Source: CAD feature listing. Evaluate the final solid. Frame: model axes, mm. A direction names the side the tool comes from. Round coordinates to 2 decimals unless told otherwise and drop trailing zeros. Loops run counter-clockwise (first coordinate to the right, second up) from the corner with the lowest first, then second, coordinate; pieces in that order, holes last. Notation, with made-up numbers: (58.5, 26) - (103.5, 26) arc R16 cw to (103.5, 49) - close; hole circle Ø11 at (89, 86.25). An arc over 180 degrees is marked (long way). One line per question, with ' | ' between items. Start each with the question number.
1. Ray query, line 1 (X direction, y = 49.5, z = -42.5); line 2 (Z direction, x = -52.5, y = 27.5); line 3 (Z direction, x = -27, y = 32.5). Return the intervals inside material, ascending.
2. Cut plane D-D (y = 68.5). Return loops of the section in (x, z).
3. Mould query, pull axis X, two halves, no side actions, for faces 1 (the flat face through (-1, 28, 45)), 2 (the cylindrical face through (-53.7, 27, 43.4)), 3 (the flat face through (0.7, 69.873, -42.465)). Classes: pulls with the +X half, pulls with the -X half, needs draft (parallel to the pull), parting line crosses it, or undercut.
4. Access query for faces 4 (the flat face through (-55, 27, -1)), 5 (the flat face through (-53, -19, 29)), 6 (the flat face through (50, 17, -1)), 7 (the flat face through (53, 57.5, 1)). Directions: +Z, -Z, +X, -X, +Y, -Y. A direction counts if a zero-diameter tool reaches every point of the face in a straight line with its end or side. Return the directions, or none.
5. Cut plane A-A (x = -52.5). Return loops of the section in (y, z), then the cut area to 3 significant figures.
6. Cut plane B-B (z = 17.5). Return loops of the section in (x, y), then the cut area to 3 significant figures.
7. Pin query (flat end, axial travel): pin 1 (4 mm diameter, centred on x = 53.5, z = 10, fed in from +Y); pin 2 (5.5 mm diameter, centred on x = -52, z = -3.5, fed in from -Y); pin 3 (1.7 mm diameter, centred on y = 59, z = -43.5, fed in from +X); pin 4 (5 mm diameter, centred on x = 52.5, z = 42.5, fed in from -Y). Return the tip coordinate at first contact, or that it passes through.
8. Cut plane C-C (y = -18). Return loops of the section in (x, z), then the cut area to 3 significant figures.
```python
from build123d import *

# Parameters (mm, degrees)
SKETCH1_W                = 100
SKETCH1_H                = 5
BOSS_EXTRUDE3_DEPTH      = 80
BOSS_EXTRUDE3_DEPTH_BACK = 24.960779397
SKETCH2_R                = 1.5
CUT_EXTRUDE1_DEPTH       = 80
SKETCH3_R                = 1.5
CUT_EXTRUDE2_DEPTH       = 80
SKETCH4_R                = 1.5
CUT_EXTRUDE3_DEPTH       = 80
SKETCH5_R                = 1.5
CUT_EXTRUDE4_DEPTH       = 80
CUT_EXTRUDE5_DEPTH       = 90
SKETCH7_W                = 90
SKETCH7_H                = 2.5
CUT_EXTRUDE7_DEPTH       = 5
CUT_EXTRUDE8_DEPTH       = 90
CUT_EXTRUDE11_DEPTH      = 90
SKETCH4_3_R              = 1.5
CUT_EXTRUDE17_DEPTH      = 105
SKETCH5_3_R              = 1.5
CUT_EXTRUDE18_DEPTH      = 105
SKETCH3_3_R              = 1.5
CUT_EXTRUDE19_DEPTH      = 105
SKETCH2_3_R              = 1.5
CUT_EXTRUDE20_DEPTH      = 105
SKETCH20_W               = 58
SKETCH20_H               = 13
CUT_EXTRUDE21_DEPTH      = 5


with BuildPart() as part:
    # Sketch1 → Boss-Extrude3 (new body, two sides)
    with BuildSketch(Plane(origin=(0, 0, 0), x_dir=(1, 0, 0), z_dir=(0, 1, 0))) as boss_extrude3_sk:
        with Locations((0, 42.5)):
            Rectangle(SKETCH1_W, SKETCH1_H)
        Polygon((-50, 45), (-55, 45), (-55, -45), (-50, -45), (-50, -40), (-50, 40), align=None)
        Polygon((55, 45), (50, 45), (50, 40), (50, -40), (50, -45), (55, -45), align=None)
        with Locations((0, -42.5)):
            Rectangle(SKETCH1_W, SKETCH1_H)
    extrude(amount=BOSS_EXTRUDE3_DEPTH)
    extrude(boss_extrude3_sk.sketch, amount=-BOSS_EXTRUDE3_DEPTH_BACK)

    # Sketch2 → Cut-Extrude1 (cut)
    with BuildSketch(Plane(origin=(0, 80, 0), x_dir=(1, 0, 0), z_dir=(0, 1, 0))):
        with Locations((-52.5, 42.5)):
            Circle(SKETCH2_R)
    extrude(amount=-CUT_EXTRUDE1_DEPTH, mode=Mode.SUBTRACT)

    # Sketch3 → Cut-Extrude2 (cut)
    with BuildSketch(Plane(origin=(0, 80, 0), x_dir=(1, 0, 0), z_dir=(0, 1, 0))):
        with Locations((52.5, 42.5)):
            Circle(SKETCH3_R)
    extrude(amount=-CUT_EXTRUDE2_DEPTH, mode=Mode.SUBTRACT)

    # Sketch4 → Cut-Extrude3 (cut)
    with BuildSketch(Plane(origin=(0, 80, 0), x_dir=(1, 0, 0), z_dir=(0, 1, 0))):
        with Locations((-52.5, -42.5)):
            Circle(SKETCH4_R)
    extrude(amount=-CUT_EXTRUDE3_DEPTH, mode=Mode.SUBTRACT)

    # Sketch5 → Cut-Extrude4 (cut)
    with BuildSketch(Plane(origin=(0, 80, 0), x_dir=(1, 0, 0), z_dir=(0, 1, 0))):
        with Locations((52.5, -42.5)):
            Circle(SKETCH5_R)
    extrude(amount=-CUT_EXTRUDE4_DEPTH, mode=Mode.SUBTRACT)

    # Sketch6 → Cut-Extrude5 (cut)
    with BuildSketch(Plane.XY.offset(45)):
        Polygon((-55, 80), (55, 80), (55, 60), align=None)
    extrude(amount=-CUT_EXTRUDE5_DEPTH, mode=Mode.SUBTRACT)

    # Sketch7 → Cut-Extrude7 (cut)
    with BuildSketch(Plane(origin=(55, 0, 0), x_dir=(0, 0, -1), z_dir=(1, 0, 0))):
        with Locations((0, 58.75)):
            Rectangle(SKETCH7_W, SKETCH7_H)
    extrude(amount=-CUT_EXTRUDE7_DEPTH, mode=Mode.SUBTRACT)

    # Sketch8 → Cut-Extrude8 (cut)
    with BuildSketch(Plane.XY.offset(45)):
        Polygon((50, 60), (55, 60), (50, 60.909090909), align=None)
    extrude(amount=-CUT_EXTRUDE8_DEPTH, mode=Mode.SUBTRACT)

    # Sketch9 → Cut-Extrude11 (cut)
    with BuildSketch(Plane.XY.offset(45)):
        Polygon((-55, 80), (-55, 77.5), (-50, 77.5), (-50, 79.090909091), align=None)
    extrude(amount=-CUT_EXTRUDE11_DEPTH, mode=Mode.SUBTRACT)

    # Sketch4_3 → Cut-Extrude17 (cut)
    with BuildSketch(Plane(origin=(0, 80, 0), x_dir=(1, 0, 0), z_dir=(0, 1, 0))):
        with Locations((-52.5, -42.5)):
            Circle(SKETCH4_3_R)
    extrude(amount=-CUT_EXTRUDE17_DEPTH, mode=Mode.SUBTRACT)

    # Sketch5_3 → Cut-Extrude18 (cut)
    with BuildSketch(Plane(origin=(0, 80, 0), x_dir=(1, 0, 0), z_dir=(0, 1, 0))):
        with Locations((52.5, -42.5)):
            Circle(SKETCH5_3_R)
    extrude(amount=-CUT_EXTRUDE18_DEPTH, mode=Mode.SUBTRACT)

    # Sketch3_3 → Cut-Extrude19 (cut)
    with BuildSketch(Plane(origin=(0, 80, 0), x_dir=(1, 0, 0), z_dir=(0, 1, 0))):
        with Locations((52.5, 42.5)):
            Circle(SKETCH3_3_R)
    extrude(amount=-CUT_EXTRUDE19_DEPTH, mode=Mode.SUBTRACT)

    # Sketch2_3 → Cut-Extrude20 (cut)
    with BuildSketch(Plane(origin=(0, 80, 0), x_dir=(1, 0, 0), z_dir=(0, 1, 0))):
        with Locations((-52.5, 42.5)):
            Circle(SKETCH2_3_R)
    extrude(amount=-CUT_EXTRUDE20_DEPTH, mode=Mode.SUBTRACT)

    # Sketch20 → Cut-Extrude21 (cut)
    with BuildSketch(Plane.ZY.offset(55)):
        with Locations((0, -18.460779397)):
            Rectangle(SKETCH20_W, SKETCH20_H)
    extrude(amount=-CUT_EXTRUDE21_DEPTH, mode=Mode.SUBTRACT)


solid = part.part
```
Answers follow:
1) line 1: x = -55 to -54, -51 to 51, 54 to 55 | line 2: z = -45 to -44, -41 to 41, 44 to 45 | line 3: z = -45 to -40, 40 to 45
2) outline: (-55, -45) - (8.25, -45) - (8.25, -40) - (-50, -40) - (-50, 40) - (8.25, 40) - (8.25, 45) - (-55, 45) - close; hole circle Ø3 at (-52.5, -42.5); hole circle Ø3 at (-52.5, 42.5)
3) face 1: needs draft | face 2: undercut | face 3: pulls with the +X half
4) face 4: +Z, -Z, -X, +Y, -Y | face 5: -X, -Y | face 6: +Y, -Y | face 7: +Z, -Z, +X, +Y
5) outline: (-24.96, -45) - (77.5, -45) - (77.5, -44) - (-24.96, -44) - close; (-24.96, -41) - (77.5, -41) - (77.5, 41) - (-24.96, 41) - (-24.96, 29) - (-11.96, 29) - (-11.96, -29) - (-24.96, -29) - close; (-24.96, 44) - (77.5, 44) - (77.5, 45) - (-24.96, 45) - close | area: 7,850 mm2
6) outline: (-55, -11.96) - (-50, -11.96) - (-50, 77.5) - (-55, 77.5) - close; (50, -24.96) - (55, -24.96) - (55, 57.5) - (50, 57.5) - close | area: 860 mm2
7) pin 1: stops at y = 57.5 | pin 2: stops at y = -11.96 | pin 3: stops at x = 50 | pin 4: stops at y = -24.96
8) outline: (-55, -45) - (55, -45) - (55, 45) - (-55, 45) - (-55, 29) - (-50, 29) - (-50, 40) - (50, 40) - (50, -40) - (-50, -40) - (-50, -29) - (-55, -29) - close; hole circle Ø3 at (-52.5, -42.5); hole circle Ø3 at (-52.5, 42.5); hole circle Ø3 at (52.5, -42.5); hole circle Ø3 at (52.5, 42.5) | area: 1,580 mm2
